Check sheet for the modelled part. Datum: model origin and axes. Units: mm. Face numbers are marked on the shaded views. A direction names the side the tool comes from. Round coordinates to 2 decimals unless told otherwise and drop trailing zeros. Loops run counter-clockwise (first coordinate to the right, second up) from the corner with the lowest first, then second, coordinate; pieces in that order, holes last. Notation, with made-up numbers: (-15.75, -28) -> (4.25, -28) arc R33 ccw to (4.25, 4) -> close; hole circle Ø6 at (38, 32). An arc over 180 degrees is marked (long way). Return JSON: item names as keys, results as strings.
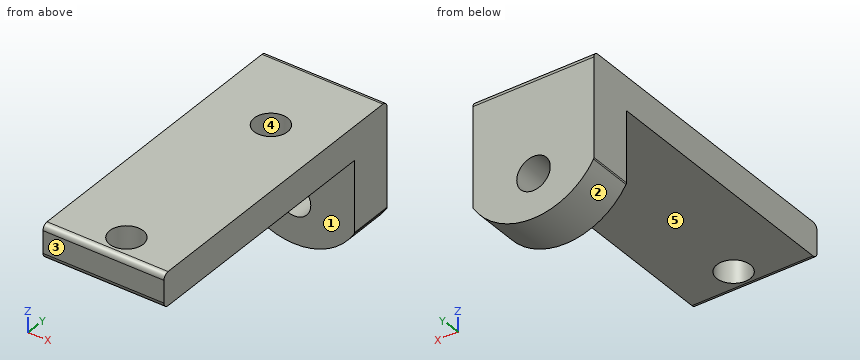
from build123d import *

# Parameters (mm, degrees)
ESBO_O2_R                = 1.5
RESSALTO_EXTRUS_O1_DEPTH = 3
ESBO_O3_R                = 1.5
RESSALTO_EXTRUS_O2_DEPTH = 4
CORTE_EXTRUS_O1_DEPTH    = 800
FILETE3_R                = 0.5
FILETE4_R                = 0.25
FILETE5_R                = 0.25
FILETE6_R                = 0.5


with BuildPart() as part:
    # Esboço2 → Ressalto-extrusão1 (new body)
    with BuildSketch(Plane.XY):
        Polygon((18.673142098, 27.45587681), (18.673142098, 15.094242614), (18.673142098, 10.125059712), (7.844942761, 10.125059712), (7.844942761, 33.593343284), (18.673142098, 33.593343284), align=None)
        with Locations((13.673142098, 30.175059712)):
            Circle(ESBO_O2_R, mode=Mode.SUBTRACT)
        with Locations((13.673142098, 12.375059712)):
            Circle(ESBO_O2_R, mode=Mode.SUBTRACT)
    extrude(amount=RESSALTO_EXTRUS_O1_DEPTH)

    # Esboço3 → Ressalto-extrusão2 (add)
    with BuildSketch(Plane(origin=(0, 33.593343284, 0), x_dir=(1, 0, 0), z_dir=(0, 1, 0))):
        with BuildLine():
            Line((7.844942761, 0), (7.844942761, -3))
            Line((7.844942761, -3), (18.673142098, -3))
            Line((18.673142098, -3), (18.673142098, 0))
            ThreePointArc((18.673142098, 0), (13.25904243, 9.495487225), (7.844942761, 0))
        make_face()
        with Locations((13.25904243, 5.554613856)):
            Circle(ESBO_O3_R, mode=Mode.SUBTRACT)
    extrude(amount=RESSALTO_EXTRUS_O2_DEPTH)

    # Esboço4 → Corte-extrusão1 (cut)
    with BuildSketch(Plane(origin=(0, 0, 0), x_dir=(1, 0, 0), z_dir=(0, 1, 0))):
        with BuildLine():
            Line((7.844942761, 0), (7.844942761, 6.408497108))
            ThreePointArc((7.844942761, 6.408497108), (6.967803758, 3.204248554), (7.844942761, 0))
        make_face()
        with BuildLine():
            Line((18.673142098, 0), (18.673142098, 6.408497108))
            ThreePointArc((18.673142098, 6.408497108), (19.550281101, 3.204248554), (18.673142098, 0))
        make_face()
    extrude(amount=CORTE_EXTRUS_O1_DEPTH, mode=Mode.SUBTRACT)

    # Filete3
    filete3_edges = [part.edges().sort_by_distance(p)[0] for p in [
        (13.25904243, 37.593343284, 3),
    ]]
    fillet(filete3_edges, radius=FILETE3_R)

    # Filete4
    filete4_edges = [part.edges().sort_by_distance(p)[0] for p in [
        (18.673142098, 35.593343284, -6.408497108),
    ]]
    fillet(filete4_edges, radius=FILETE4_R)

    # Filete5
    filete5_edges = [part.edges().sort_by_distance(p)[0] for p in [
        (7.844942761, 35.593343284, -6.408497108),
    ]]
    fillet(filete5_edges, radius=FILETE5_R)

    # Filete6
    filete6_edges = [part.edges().sort_by_distance(p)[0] for p in [
        (13.25904243, 10.125059712, 3),
        (13.25904243, 10.125059712, 0),
    ]]
    fillet(filete6_edges, radius=FILETE6_R)


solid = part.part
Q1. Material ranges on line 1 (Z direction, x = 11.5, y = 23.25); line 2 (Y direction, x = 16.25, z = -4.75); line 3 (Z direction, x = 12.5, y = 34), recorded low to high.
Results list:
{"line 1": "0 to 3", "line 2": "33.59 to 37.59", "line 3": "-9.45 to -6.85, -4.26 to 3"}
Q2. Tool access check on the marked faces 1 and 2. Record the directions out of +Z, -Z, +X, -X, +Y, -Y that give a thin tool (end or side, any length) a straight path to the whole face; none if there is none.
Results list:
{"face 1": "-Z, +X, -X, -Y", "face 2": "-Z, +Y, -Y"}
Q3. Section check C-C (z = -5). Record the boundary of the cut face in (x, y), then the cut area to 3 significant figures.
Results list:
{"outline": "(7.84, 33.59) -> (11.87, 33.59) -> (11.87, 37.59) -> (7.84, 37.59) -> close; (14.65, 33.59) -> (18.67, 33.59) -> (18.67, 37.59) -> (14.65, 37.59) -> close", "area": "32.2 mm^2"}
Q4. Section check A-A (y = 13.5). Record the boundary of the cut face in (x, z), then the cut area to 3 significant figures.
Results list:
{"outline": "(7.84, 0) -> (12.68, 0) -> (12.68, 3) -> (7.84, 3) -> close; (14.67, 0) -> (18.67, 0) -> (18.67, 3) -> (14.67, 3) -> close", "area": "26.5 mm^2"}
Q5. Go/stop test with a flat-tipped pin: pin 1 (3 mm diameter, centred on x = 13, y = 27.5, fed in from -Z). Record where the tip stops, or that it passes through.
Results list:
{"pin 1": "z = 0"}
Q6. Draft check along Y on the marked faces 3, 4 and 5. Enter one of: released by +Y, released by -Y, zero draft, split by the parting line, or undercut.
Results list:
{"face 3": "released by -Y", "face 4": "undercut", "face 5": "zero draft"}
Q7. Section check D-D (y = 35). Record the boundary of the cut face in (x, z), then the cut area to 3 significant figures.
Results list:
{"outline": "(7.84, -6.34) arc R0.25 ccw to (7.88, -6.47) arc R6.29 ccw to (18.64, -6.47) arc R0.25 ccw to (18.67, -6.34) -> (18.67, 3) -> (7.84, 3) -> close; hole circle Ø3 at (13.26, -5.55)", "area": "118 mm^2"}
Q8. Section check B-B (x = 14.5). Record the boundary of the cut face in (y, z), then the cut area to 3 significant figures.
Results list:
{"outline": "(10.13, 0.5) arc R0.5 ccw to (10.63, 0) -> (11.12, 0) -> (11.12, 3) -> (10.63, 3) arc R0.5 ccw to (10.13, 2.5) -> close; (13.63, 0) -> (28.92, 0) -> (28.92, 3) -> (13.63, 3) -> close; (31.43, 0) -> (33.59, 0) -> (33.59, -4.71) -> (37.59, -4.71) -> (37.59, 2.5) arc R0.5 ccw to (37.09, 3) -> (31.43, 3) -> close; (33.59, -9.37) -> (37.59, -9.37) -> (37.59, -6.4) -> (33.59, -6.4) -> close", "area": "98.0 mm^2"}
